Read the model definition and answer for the solid it produces. Units are mm, in the model's axes. A direction names the side the tool comes from. Give positions to 0.01 mm unless a question says otherwise; leave off trailing zeros. Order: outer loops, then holes, each group sorted by start corner. A loop starts at its lowest first (then second) coordinate and runs counter-clockwise, first axis right, second up.
Autodesk Inventor part; units mm, degrees
ref_plane "YZ Plane" through (0, 0, 0) normal (1, 0, 0) x (0, 1, 0)
ref_plane "XZ Plane" through (0, 0, 0) normal (0, 1, 0) x (-1, 0, 0)
ref_plane "XY Plane" through (0, 0, 0) normal (0, 0, 1) x (1, 0, 0)
sketch "Sketch1" plane through (0, 0, 0) normal (0, 1, 0) x (-1, 0, 0)
  line L0 (0, 0) -> (-25.32, 0)
  line L1 (-25.32, 0) -> (-25.32, -13)
  line L2 (-25.32, -13) -> (0, -13)
  line L3 (0, -13) -> (0, 0)
  dimension "d0" = 25.32
  dimension "d1" = 13
extrude "Extrusion1" add sketch "Sketch1" along normal blind 5
sketch "Sketch2" plane through (25.32, 0, 0) normal (1, 0, 0) x (0, 0, -1)
  line L0 (0, 0) -> (13, 0)
  line L1 (13, 0) -> (13, 21.3)
  line L2 (13, 21.3) -> (0, 21.3)
  line L3 (0, 21.3) -> (0, 0)
  dimension "d4" = 13
  dimension "d5" = 21.3
extrude "Extrusion2" add sketch "Sketch2" along normal blind 7
sketch "Sketch3" plane through (0, 0, 0) normal (0, -1, 0) x (1, 0, 0)
  line L0 (25.32, -13) -> (0, -13)
  line L1 (25.32, -8.0084) -> (25.32, -13)
  line L2 (25.32, -13) -> (25.32, -23) construction
  line L3 (25.32, -23) -> (20.12, -23) construction
  line L4 (20.12, -23) -> (25.32, -13)
  line L5 (20.12, -23) -> (5.2, -23)
  line L6 (0, -23) -> (5.2, -23)
  line L7 (5.2, -23) -> (0, -13)
  line L8 (0, -13) -> (5.2, -23)
  point P0 (0, 0)
  dimension "d8" = 10
  dimension "d9" = 5.2
  dimension "d10" = 5.2
extrude "Extrusion3" add sketch "Sketch3" against normal blind 5
sketch "Sketch4" plane through (0, 0, 0) normal (0, -1, 0) x (1, 0, 0)
  line L0 (20.12, -23) -> (25.32, -13)
  line L1 (20.12, -23) -> (27.32, -23)
  line L2 (25.32, -13) -> (32.32, -13)
  line L3 (32.32, -13) -> (27.32, -23)
  point P0 (0, 0)
  dimension "d13" = 7.2
extrude "Extrusion4" add sketch "Sketch4" against normal blind 21.3
sketch "Sketch5" plane through (0, 0, 0) normal (0, -1, 0) x (1, 0, 0)
  line L0 (20.12, -23) -> (5.2, -23)
  line L1 (20.12, -23) -> (20.12, -28.9) construction
  line L2 (20.12, -28.9) -> (22.12, -28.9) construction
  line L3 (20.12, -23) -> (25.32, -13)
  line L4 (22.12, -28.9) -> (20.12, -23)
  line L5 (27.32, -23) -> (20.12, -23)
  line L6 (27.32, -23) -> (27.32, -28.9)
  line L7 (27.32, -28.9) -> (29.32, -28.9) construction
  line L8 (29.32, -28.9) -> (27.32, -23)
  line L9 (29.32, -28.9) -> (22.12, -28.9)
  line L10 (5.2, -23) -> (5.2, -28.9) construction
  line L11 (5.2, -28.9) -> (3.2, -28.9) construction
  line L12 (3.2, -28.9) -> (5.2, -23)
  line L13 (22.12, -28.9) -> (3.2, -28.9)
  point P0 (0, 0)
  dimension "d16" = 5.9
  dimension "d17" = 2
  dimension "d18" = 2
  dimension "d19" = 2
extrude "Extrusion5" add sketch "Sketch5" against normal blind 5 contours L4 L13 L12 L0
sketch "Sketch6" plane through (0, 0, 0) normal (0, -1, 0) x (1, 0, 0)
  line L0 (20.12, -23) -> (27.32, -23)
  line L1 (27.32, -23) -> (27.32, -28.9) construction
  line L2 (27.32, -28.9) -> (29.32, -28.9) construction
  line L3 (29.32, -28.9) -> (27.32, -23)
  line L4 (20.12, -23) -> (22.12, -28.9)
  line L5 (29.32, -28.9) -> (22.12, -28.9)
  point P0 (0, 0)
  dimension "d22" = 5.9
  dimension "d23" = 2
extrude "Extrusion6" add sketch "Sketch6" against normal blind 21.3
sketch "Sketch7" plane through (0, 0, 0) normal (0, -1, 0) x (1, 0, 0)
  line L0 (22.12, -28.9) -> (3.2, -28.9)
  line L1 (22.12, -28.9) -> (22.12, -31.4)
  line L2 (3.2, -28.9) -> (5.2, -23)
  line L3 (3.2, -28.9) -> (3.2, -31.4)
  line L4 (3.2, -31.4) -> (22.12, -31.4)
  point P0 (0, 0)
  dimension "d26" = 2.5
  dimension "d27" = 2.5
extrude "Extrusion7" add sketch "Sketch7" against normal blind 5
sketch "Sketch8" plane through (0, 0, 0) normal (0, -1, 0) x (1, 0, 0)
  line L0 (27.32, -23) -> (29.32, -28.9)
  line L1 (22.12, -28.9) -> (22.12, -31.4)
  line L2 (29.32, -28.9) -> (22.12, -28.9)
  line L3 (22.12, -28.9) -> (22.12, -31.4)
  line L4 (22.12, -31.4) -> (29.32, -31.4)
  line L5 (29.32, -31.4) -> (29.32, -28.9)
  point P0 (0, 0)
extrude "Extrusion8" add sketch "Sketch8" against normal blind 21.3
sketch "Sketch9" plane through (0, 0, 0) normal (0, -1, 0) x (1, 0, 0)
  line L0 (22.12, -31.4) -> (3.2, -31.4)
  line L1 (3.2, -31.4) -> (22.12, -31.4)
  line L2 (22.12, -31.4) -> (22.12, -39.7)
  line L3 (22.12, -39.7) -> (3.2, -39.7)
  line L4 (3.2, -39.7) -> (3.2, -31.4)
  point P0 (0, 0)
  dimension "d32" = 18.92
  dimension "d33" = 8.3
extrude "Extrusion9" add sketch "Sketch9" against normal blind 21.3
sketch "Sketch10" plane through (0, 0, 0) normal (0, -1, 0) x (1, 0, 0)
  line L0 (22.12, -31.4) -> (29.32, -31.4)
  line L1 (22.12, -31.4) -> (22.12, -39.7)
  line L2 (29.32, -31.4) -> (22.12, -39.7)
  point P0 (0, 0)
extrude "Extrusion10" add sketch "Sketch10" against normal blind 21.3
sketch "Sketch11" plane through (3.2, 0, -39.7) normal (0, 0, -1) x (-1, 0, 0)
  line L0 (0, 5) -> (-2, 5)
  line L1 (0, 5) -> (-18.878, 5) construction
  line L2 (0, 21.3) -> (-18.92, 21.3)
  line L3 (-9.46, 21.3) -> (-9.439, 5) construction
  line L4 (-9.4495, 13.15) -> (0, 13.1622) construction
  line L5 (0, 0) -> (0, 21.3)
  circle A0 centre (-9.4495, 13.15) radius 6.625
  point P0 (3.2, 0)
  dimension "d38" = 13.25
extrude "Extrusion11" cut sketch "Sketch11" against normal blind 21.3
sketch "Sketch12" plane through (25.32, 21.3, 0) normal (0, 1, 0) x (1, 0, 0)
  line L0 (7, 13) -> (2, 23)
  line L1 (4, 31.4) -> (4, 28.9)
  line L2 (7, 13) -> (4, 31.4)
  line L3 (2, 23) -> (4, 28.9)
  line L4 (2, 23) -> (4, 28.9)
  line L5 (4, 28.9) -> (4, 31.4)
  line L6 (7, 13) -> (2, 23)
  point P0 (-25.32, 0)
extrude "Extrusion12" add sketch "Sketch12" against normal blind 21.3
sketch "Sketch13" plane through (25.32, 21.3, 0) normal (0, 1, 0) x (1, 0, 0)
  line L0 (4, 31.4) -> (7, 13)
  line L1 (7, 13) -> (7, 31.4) construction
  line L2 (4, 31.4) -> (7, 27.9417)
  line L3 (4, 31.4) -> (-3.2, 39.7)
  line L4 (7, 27.9417) -> (7, 13)
  line L5 (7, 13) -> (4, 31.4)
  point P0 (-25.32, 0)
extrude "Extrusion13" add sketch "Sketch13" against normal blind 21.3
ref_plane "Work Plane1" through (12.66, 5, 0) normal (1, 0, 0) x (0, 1, 0)
mirror "Mirror1" about plane through (12.66, 5, 0) normal (1, 0, 0)
sketch "Sketch16" plane through (25.32, 5, 0) normal (0, 0, 1) x (1, 0, 0)
  line L0 (-20.12, 0) -> (-25.32, 0)
  line L1 (-25.32, 0) -> (-25.32, -2) construction
  line L2 (-25.32, -2) -> (-27.32, -2)
  line L3 (-27.32, -2) -> (-27.32, 16.3)
  line L4 (-25.32, 16.3) -> (-32.32, 16.3)
  line L5 (0, 0) -> (2, 0) construction
  line L6 (2, 0) -> (2, -2)
  line L7 (2, -2) -> (-25.32, -2)
  line L8 (2, 0) -> (2, 16.3)
  line L9 (-27.32, 16.3) -> (-32.32, 16.3)
  line L10 (-32.32, 16.3) -> (-32.32, -5)
  line L11 (-32.32, 16.3) -> (-32.32, -5)
  line L12 (-32.32, -5) -> (7, -5)
  line L13 (7, 16.3) -> (7, -5)
  line L14 (7, -5) -> (7, 16.3)
  line L15 (7, 16.3) -> (2, 16.3)
  line L16 (0, 16.3) -> (7, 16.3)
  point P0 (-25.32, -5)
  dimension "d45" = 2
  dimension "d46" = 2
  dimension "d47" = 2
  dimension "d48" = 2
extrude "Extrusion14" add sketch "Sketch16" along normal blind 19.2
sketch "Sketch22" plane through (-7, 0, -27.9417) normal (-1, 0, 0) x (0, 0, 1)
  line L0 (-11.7583, 0) -> (0, 0)
  line L1 (0, 0) -> (8, 0)
  line L2 (8, 0) -> (8, -8)
  line L3 (8, -8) -> (0, -8)
  line L4 (0, -8) -> (0, 0)
  line L5 (47.1417, 0) -> (0, 0)
  line L6 (47.1417, 0) -> (39.1417, 0)
  line L7 (39.1417, 0) -> (39.1417, -8)
  line L8 (39.1417, -8) -> (47.1417, -8)
  line L9 (47.1417, -8) -> (47.1417, 0)
  line L10 (0, -4) -> (47.1417, -4) construction
  line L11 (4, -8) -> (4, -4) construction
  line L12 (43.1417, -8) -> (43.1417, -4) construction
  circle A0 centre (4, -4) radius 1
  circle A1 centre (43.1417, -4) radius 1
  point P0 (27.9417, 0)
  dimension "d81" = 8
  dimension "d82" = 8
  dimension "d83" = 8
  dimension "d84" = 8
  dimension "d85" = 2
  dimension "d86" = 2
extrude "Extrusion20" add sketch "Sketch22" against normal blind 2.5
chamfer "Chamfer2" distance 2 angle 45 2 edges at (-4.5, -4, -24.9417) (-4.5, -4, 14.2)
sketch "Sketch24" plane through (25.32, 21.3, 0) normal (0, 1, 0) x (1, 0, 0)
  line L0 (-27.32, -19.2) -> (-32.32, -19.2)
  line L1 (-27.32, -19.2) -> (-32.32, -19.2)
  line L2 (-32.32, 27.9417) -> (-32.32, -19.2)
  line L3 (-32.32, -19.2) -> (-32.32, 27.9417)
  line L4 (-32.32, 27.9417) -> (-22.12, 39.7)
  line L5 (-32.32, 27.9417) -> (-22.12, 39.7)
  line L6 (-3.2, 39.7) -> (-22.12, 39.7)
  line L7 (-22.12, 39.7) -> (-3.2, 39.7)
  line L8 (-3.2, 39.7) -> (7, 27.9417)
  line L9 (7, -19.2) -> (7, 27.9417)
  line L10 (7, 27.9417) -> (7, -19.2)
  line L11 (7, -19.2) -> (2, -19.2)
  line L12 (7, -19.2) -> (2, -19.2)
  line L13 (0, 0) -> (2, 0)
  line L14 (2, -19.2) -> (2, 0)
  line L15 (2, 0) -> (0, 0)
  line L16 (0, 13) -> (0, 0)
  line L17 (0, 0) -> (0, 13)
  line L18 (-5.2, 23) -> (0, 13)
  line L19 (0, 13) -> (-5.2, 23)
  line L20 (-3.2, 28.9) -> (-5.2, 23)
  line L21 (-5.2, 23) -> (-3.2, 28.9)
  line L22 (-3.2, 28.9) -> (-3.2, 31.4)
  line L23 (-22.12, 31.4) -> (-3.2, 31.4)
  line L24 (-3.2, 31.4) -> (-22.12, 31.4)
  line L25 (-22.12, 31.4) -> (-22.12, 28.9)
  line L26 (-22.12, 31.4) -> (-22.12, 28.9)
  line L27 (-22.12, 28.9) -> (-20.12, 23)
  line L28 (-22.12, 28.9) -> (-20.12, 23)
  line L29 (-20.12, 23) -> (-25.32, 13)
  line L30 (-20.12, 23) -> (-25.32, 13)
  line L31 (-25.32, 13) -> (-25.32, 0)
  line L32 (-25.32, 13) -> (-25.32, 0)
  line L33 (-25.32, 0) -> (-27.32, 0)
  line L34 (-25.32, 0) -> (-27.32, 0)
  line L35 (-27.32, 0) -> (-27.32, -19.2)
  line L36 (-27.32, 0) -> (-27.32, -19.2)
  line L37 (-25.32, 13) -> (-25.32, 0)
  line L38 (0, 0) -> (-25.32, 0)
extrude "Extrusion22" add sketch "Sketch24" along normal blind 2 contours L0 L2 L4 L6 L8 L9 L11 L14 L13 L16 L18 L20 L22 L23 L25 L27 L29 L31 L33 L35
sketch "Sketch25" plane through (25.32, 23.3, 0) normal (0, 1, 0) x (1, 0, 0)
  line L0 (2, -19.2) -> (7, -19.2)
  line L1 (7, -19.2) -> (15, -19.2)
  line L2 (15, -19.2) -> (15, -11.2)
  line L3 (15, -11.2) -> (7, -11.2)
  line L4 (7, -11.2) -> (7, -19.2)
  line L5 (7, -19.2) -> (7, 27.9417)
  line L6 (7, 27.9417) -> (15, 27.9417)
  line L7 (15, 27.9417) -> (15, 19.9417)
  line L8 (15, 19.9417) -> (7, 19.9417)
  line L9 (7, 19.9417) -> (7, 27.9417)
  line L10 (11, -19.2) -> (11, 27.9417) construction
  line L11 (15, -15.2) -> (11, -15.2) construction
  line L12 (15, 23.9417) -> (11, 23.9417) construction
  circle A0 centre (11, -15.2) radius 1
  circle A1 centre (11, 23.9417) radius 1
  point P0 (-25.32, 0)
  dimension "d96" = 8
  dimension "d97" = 8
  dimension "d98" = 8
  dimension "d99" = 8
  dimension "d100" = 2
  dimension "d101" = 2
extrude "Extrusion23" add sketch "Sketch25" against normal blind 2
chamfer "Chamfer3" distance 2 angle 45 2 edges at (35.32, 21.3, 15.2) (35.32, 21.3, -23.9417)
sketch "Sketch26" plane through (25.32, 21.3, 0) normal (0, -1, 0) x (1, 0, 0)
  circle A0 centre (11, 15.2) radius 1
  circle A1 centre (11, 15.2) radius 3
  line L0 (15, 19.2) -> (7, 19.2)
  line L1 (7, 11.2) -> (7, 19.2)
  line L2 (7, 11.2) -> (15, 11.2)
  line L3 (15, 11.2) -> (15, 19.2)
  circle A2 centre (11, 15.2) radius 3
  circle A3 centre (11, 15.2) radius 3
  line L4 (15, 19.2) -> (7, 19.2)
  line L5 (15, 19.2) -> (7, 19.2)
  line L6 (7, 19.2) -> (7, 11.2)
  line L7 (7, 11.2) -> (15, 11.2)
  line L8 (15, 11.2) -> (15, 19.2)
  point P0 (-25.32, 0)
extrude "Extrusion24" add sketch "Sketch26" along normal blind 21.3 contours L3 L2 L1 L0
sketch "Sketch28" plane through (25.32, 21.3, 0) normal (0, -1, 0) x (1, 0, 0)
  circle A0 centre (11, -23.9417) radius 1
  circle A1 centre (11, -23.9417) radius 3
  line L0 (7, -27.9417) -> (7, -19.9417)
  line L1 (7, -27.9417) -> (15, -27.9417)
  line L2 (15, -27.9417) -> (15, -19.9417)
  line L3 (15, -19.9417) -> (7, -19.9417)
  circle A2 centre (11, -23.9417) radius 3
  circle A3 centre (11, -23.9417) radius 3
  line L4 (7, -27.9417) -> (-3.2, -39.7)
  line L5 (15, -19.9417) -> (15, -27.9417)
  line L6 (7, -27.9417) -> (15, -27.9417)
  line L7 (15, -27.9417) -> (15, -19.9417)
  line L8 (15, -19.9417) -> (7, -19.9417)
  line L9 (7, -19.9417) -> (7, -27.9417)
  point P0 (-25.32, 0)
extrude "Extrusion25" add sketch "Sketch28" along normal blind 21.3 contours L0 L3 L2 L1
sketch "Sketch29" plane through (-4.5, 0, -27.9417) normal (1, 0, 0) x (0, 0, -1)
  circle A0 centre (-43.1417, -4) radius 1
  circle A1 centre (-43.1417, -4) radius 3
  line L0 (-47.1417, 0) -> (-39.1417, 0)
  line L1 (-47.1417, 0) -> (-47.1417, -8)
  line L2 (-47.1417, -8) -> (-39.1417, -8)
  line L3 (-39.1417, -8) -> (-39.1417, 0)
  circle A2 centre (-43.1417, -4) radius 3
  circle A3 centre (-4, -4) radius 1
  circle A4 centre (-4, -4) radius 3
  line L4 (0, -8) -> (0, 0)
  line L5 (-8, 0) -> (0, 0)
  line L6 (-8, 0) -> (-8, -8)
  line L7 (-8, -8) -> (0, -8)
  circle A5 centre (-4, -4) radius 3
  line L8 (-39.1417, -8) -> (-47.1417, -8)
  line L9 (-47.1417, -8) -> (-47.1417, 0)
  line L10 (-47.1417, 0) -> (-39.1417, 0)
  line L11 (-39.1417, 0) -> (-39.1417, -8)
  line L12 (-8, -8) -> (0, -8)
  line L13 (0, -8) -> (-8, -8)
  line L14 (-8, -8) -> (-8, 0)
  line L15 (-8, 0) -> (0, 0)
  line L16 (0, 0) -> (0, -8)
  circle A6 centre (-43.1417, -4) radius 3
  circle A7 centre (-4, -4) radius 1
  circle A8 centre (-4, -4) radius 3
  point P0 (-27.9417, 0)
extrude "Extrusion26" add sketch "Sketch29" along normal blind 20 contours L0 L3 L2 L1 | L7 L6 L5 L4
properties part number "AC_wire_holder"
1) The part is cut by section A-A on y = -4. Determine the outline of the cut face in (x, z).
Final values:
outline: (-7, -27.94) - (15.5, -27.94) - (15.5, -26.94) - (-4.5, -26.94) - (-6.5, -24.94) - (-7, -24.94) - close; (-7, -22.94) - (-6.5, -22.94) - (-4.5, -20.94) - (15.5, -20.94) - (15.5, -19.94) - (-7, -19.94) - close; (-7, 11.2) - (15.5, 11.2) - (15.5, 12.2) - (-4.5, 12.2) - (-6.5, 14.2) - (-7, 14.2) - close; (-7, 16.2) - (-6.5, 16.2) - (-4.5, 18.2) - (15.5, 18.2) - (15.5, 19.2) - (-7, 19.2) - close
2) The part is cut by section B-B on z = -19. Determine the outline of the cut face in (x, y).
Final values:
outline: (-7, 0) - (32.32, 0) - (32.32, 23.3) - (22.2, 23.3) - (22.2, 5) - (3.12, 5) - (3.12, 23.3) - (-7, 23.3) - close
3) For a pull along X with two mould halves and no side action, classify faces 1 (the face through (40.32, 12, 15)), 2 (the face through (0, 14, -7)), 3 (the face through (4, -4, -19.942)) as released by +X, released by -X, zero draft, split by the parting line, or undercut.
Final values:
face 1: released by +X
face 2: undercut
face 3: zero draft
4) The part is cut by section C-C on y = 11. Count the separate pieces of the cut face and the enclosed holes in it, and give its area (3 significant figures).
Final values:
separate pieces: 2
enclosed holes: 2
area: 923 mm2
5) Consider L1, parallel to Z at x = 36, y = 17; L2, parallel to Z at x = 6, y = -4; L3, parallel to X at y = 23, z = 15. Determine where each line is inside the solid, lowest interval first.
Final values:
L1: z = -27.94 to -26.92, -20.96 to -19.94, 11.2 to 12.22, 18.18 to 19.2
L2: z = -27.94 to -26.94, -20.94 to -19.94, 11.2 to 12.2, 18.2 to 19.2
L3: x = -7 to -2, 27.32 to 35.04, 37.6 to 40.32
6) Given pin 1 (2 mm diameter, centred on y = -3, z = 12, fed in from +X); pin 2 (6.5 mm diameter, centred on y = 12, z = -9, fed in from +X); pin 3 (9 mm diameter, centred on x = 34.5, y = 17, fed in from -Z), each flat-ended and moving along its own axis, determine where each tip first touches the part or whether it passes through.
Final values:
pin 1: stops at x = 15.5
pin 2: stops at x = 32.32
pin 3: stops at z = -30.62
7) The part is cut by section D-D on x = 10. Determine the outline of the cut face in (y, z), and give its area (3 significant figures).
Final values:
outline: (-8, -27.94) - (0, -27.94) - (0, -39.7) - (7.09, -39.7) - (7.09, -31.4) - (5, -31.4) - (5, 0) - (3, 0) - (3, 19.2) - (-8, 19.2) - (-8, 11.2) - (0, 11.2) - (0, -19.94) - (-8, -19.94) - close; (19.21, -39.7) - (23.3, -39.7) - (23.3, -31.4) - (19.21, -31.4) - close; hole circle Ø6 at (-4, -23.94); hole circle Ø6 at (-4, 15.2)
area: 379 mm2
8) A tool of negligible diameter and unlimited length cuts with its end or side. For faces 4 (the face through (22.684, 14.022, -18.07)), 5 (the face through (36, 12, -19.942)), 6 (the face through (4, -4, -27.942)), 7 (the face through (3.2, 14, -30)), 8 (the face through (4, -4, 11.2)), from which of +Z, -Z, +X, -X, +Y, -Y can it reach the whole face along a straight path? Write none if from no direction.
Final values:
face 4: +Z, +Y
face 5: +X, +Y, -Y
face 6: -Z, +X, -X, -Y
face 7: +Y
face 8: +X, -X, -Y
